Check sheet for the modelled part. Datum: model origin and axes. Units: mm. Give positions to 0.01 mm unless a question says otherwise; leave off trailing zeros. Order: outer loops, then holes, each group sorted by start corner. A loop starts at its lowest first (then second) coordinate and runs counter-clockwise, first axis right, second up. Notation, with made-up numbers: (-29.75, 78) -> (17.25, 78) arc R18 cw to (17.25, 88) -> close; hole circle Ø1 at (-34, 76). An arc over 180 degrees is marked (long way). Answer in a Markdown table with one row per item. Add a question column.
(1) Go/stop test with a flat-tipped pin: pin 1 (1 mm diameter, centred on y = -133.5, z = -176.5, fed in from -X). Record where the tip stops, or that it passes through.
(2) Thickness scan on L1, parallel to Y at x = 0.05, z = -25.5; L2, parallel to Z at x = 0.05, y = -117; L3, parallel to Y at x = 0.05, z = -346. Record the ranges inside material, lowest first. Write a range as [from, to].
(3) Cross-section at A-A (y = -143.5). Record the cut outline in (x, z).
```python
from build123d import *

# Parameters (mm, degrees)
BOSS_EXTRUDE1_DEPTH = 0.127


with BuildPart() as part:
    # Sketch1 → Boss-Extrude1 (new body)
    with BuildSketch(Plane(origin=(0, 0, 0), x_dir=(0, 0, -1), z_dir=(1, 0, 0))):
        with BuildLine():
            Line((734.40708933, 124.676146582), (733.357043785, 29.761237691))
            Line((733.357043785, 29.761237691), (328.770751491, -205.523937709))
            Line((328.770751491, -205.523937709), (-328.770779224, -205.523937708))
            Line((-328.770779224, -205.523937708), (-733.357071518, 29.761237693))
            Line((-733.357071518, 29.761237693), (-734.407163707, 124.676062292))
            add(Edge.make_bspline(
                [(-1.3866e-05, -78.523920986), (-367.203581261, -78.523944347), (-734.407163707, 124.676062292)],
                knots=[0, 0, 0, 1, 1, 1], degree=2))
            add(Edge.make_bspline(
                [(-1.3866e-05, -78.523920986), (367.203545257, -78.523897625), (734.40708933, 124.676146582)],
                knots=[0, 0, 0, 1, 1, 1], degree=2))
        make_face()
    extrude(amount=BOSS_EXTRUDE1_DEPTH)


solid = part.part
```
Answer below:
| question | item | result |
|---|---|---|
| 1 | pin 1 | stops at x = 0 |
| 2 | L1 | y = [-205.52, -78.28] |
| 2 | L2 | z = [-480.99, 480.99] |
| 2 | L3 | y = [-195.5, -33.42] |
| 3 | outline | (0, -435.42) -> (0.13, -435.42) -> (0.13, 435.42) -> (0, 435.42) -> close |
